Here's how the part is built. I have some questions about the finished solid (model axes, mm). Coordinates: 2 decimals unless noted, no trailing zeros. Write each loop counter-clockwise with the first axis right and the second up, starting at its lowest first coordinate (ties: lowest second). Pieces come first, ordered by that corner, then holes. Notation, with made-up numbers: (-21.5, 25) -> (22.5, 25) arc R30 cw to (22.5, 63) -> close; hole circle Ø6 at (-19.5, -34.75). An arc over 180 degrees is marked (long way). Use a Markdown table: item, result. Add a question column.
```python
from build123d import *

# Parameters (mm, degrees)
SKETCH_W   = 20
SKETCH_H   = 20
SKETCH_W_2 = 180
SKETCH_H_2 = 5.214788
SKETCH_W_3 = 5
SKETCH_H_3 = 180
SKETCH_H_4 = 5
PAD_DEPTH  = 1


with BuildPart() as part:
    # Sketch (on XY_Plane of Origin) → Pad (new body)
    with BuildSketch(Plane.XY):
        with Locations((-100, 100)):
            Rectangle(SKETCH_W, SKETCH_H)
        with Locations((-100, -100)):
            Rectangle(SKETCH_W, SKETCH_H)
        with Locations((100, -100)):
            Rectangle(SKETCH_W, SKETCH_H)
        with Locations((100, 100)):
            Rectangle(SKETCH_W, SKETCH_H)
        with Locations((0, 99.892606)):
            Rectangle(SKETCH_W_2, SKETCH_H_2)
        with Locations((-100, 0)):
            Rectangle(SKETCH_W_3, SKETCH_H_3)
        with Locations((0, -100)):
            Rectangle(SKETCH_W_2, SKETCH_H_4)
        with Locations((100, 0)):
            Rectangle(SKETCH_W_3, SKETCH_H_3)
    extrude(amount=PAD_DEPTH)


solid = part.part
```
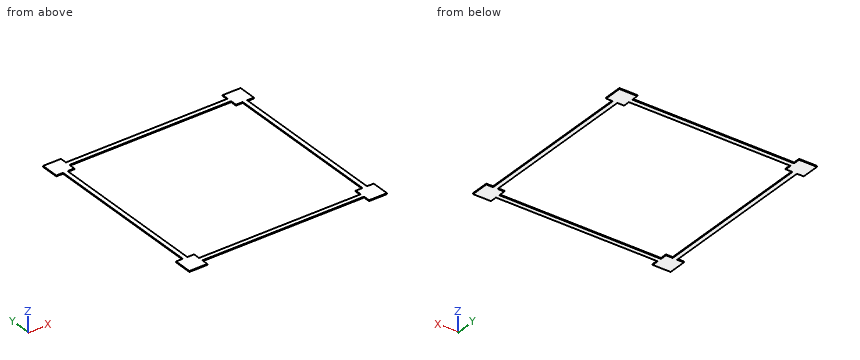
Q1. Will this pin go through, and if not, where does the flat tip stop? pin 1 (0.5 mm diameter, centred on x = 45, z = 0.5, fed in from -Y).
Q2. Suppose I cut it at B-B, the plane x = 55. Write out the boundary of the cut face in (y, z), and give its area (3 significant figures).
Q3. Suppose I cut it at A-A, the plane y = -81. Write out the boundary of the cut face in (x, z).
Q4. Please list where these lines run through material, in increasing order: line 1 (X direction, y = 10, z = 0.8); line 2 (X direction, y = 91.5, z = 0.5); line 3 (Y direction, x = -21.5, z = 0.75).
Answer key:
| question | item | result |
|---|---|---|
| 1 | pin 1 | stops at y = -102.5 |
| 2 | outline | (-102.5, 0) -> (-97.5, 0) -> (-97.5, 1) -> (-102.5, 1) -> close; (97.29, 0) -> (102.5, 0) -> (102.5, 1) -> (97.29, 1) -> close |
| 2 | area | 10.2 mm^2 |
| 3 | outline | (-102.5, 0) -> (-97.5, 0) -> (-97.5, 1) -> (-102.5, 1) -> close; (97.5, 0) -> (102.5, 0) -> (102.5, 1) -> (97.5, 1) -> close |
| 4 | line 1 | x = -102.5 to -97.5, 97.5 to 102.5 |
| 4 | line 2 | x = -110 to -90, 90 to 110 |
| 4 | line 3 | y = -102.5 to -97.5, 97.29 to 102.5 |
